```python
from build123d import *

# Parameters (mm, degrees)
F1_DEPTH = 19.05
F2_W     = 152.4
F2_H     = 19.05
F3_DEPTH = 19.051
F4_R     = 12.7
F5_DEPTH = 19.051


with BuildPart() as f1:
    # F0 (on Top) → F1 (new body)
    with BuildSketch(Plane.XY):
        Polygon((341.488764, -53.718452), (318.628764, -53.718452), (318.628764, -2.918452), (341.488764, -2.918452), (341.488764, 30.101548), (-268.111236, 30.101548), (-268.111236, -2.918452), (-245.251236, -2.918452), (-245.251236, -53.718452), (-268.111236, -53.718452), (-268.111236, -86.738452), (-268.111236, -105.788452), (341.488764, -105.788452), (341.488764, -86.738452), align=None)
    extrude(amount=F1_DEPTH)

    # F2 (on face) → F3 (cut, through all)
    with BuildSketch(Plane.XY.offset(19.05)):
        with Locations((-115.711236, -96.263452)):
            Rectangle(F2_W, F2_H)
        with Locations((189.088764, -96.263452)):
            Rectangle(F2_W, F2_H)
    extrude(amount=-F3_DEPTH, mode=Mode.SUBTRACT)

    # F4 (on face) → F5 (cut, through all)
    with BuildSketch(Plane.XY.offset(19.05)):
        with Locations((189.088764, -28.318452)):
            Circle(F4_R)
        with Locations((-115.711236, -28.318452)):
            Circle(F4_R)
    extrude(amount=-F5_DEPTH, mode=Mode.SUBTRACT)


solid = f1.part
```
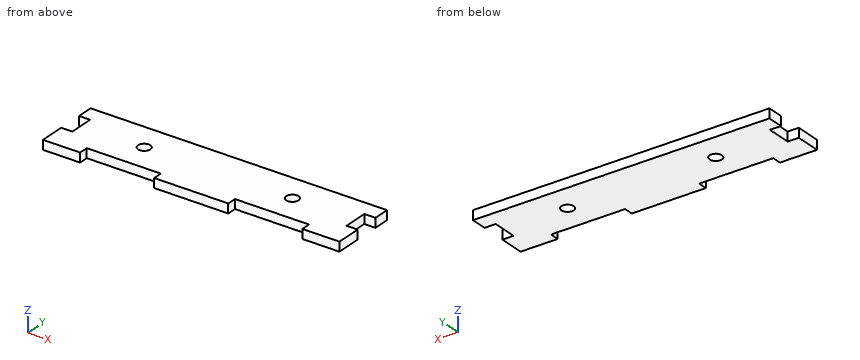
Part model, mm, in its own coordinate system. Coordinates: 2 decimals unless noted, no trailing zeros. Write each loop counter-clockwise with the first axis right and the second up, starting at its lowest first coordinate (ties: lowest second). Pieces come first, ordered by that corner, then holes.
Item 1: Slice it at A-A (x = 190). Write the cut outline in (y, z), and give its area (3 significant figures).
Item 2: Pin check, flat tips, straight feed: pin 1 (5.5 mm diameter, centred on x = -91.5, z = 10.5, fed in from -Y); pin 2 (6 mm diameter, centred on y = -10, z = 16.5, fed in from -X); pin 3 (23 mm diameter, centred on x = -115.71, y = -28.32, fed in from -Z). Stop position of each tip, or through.
Item 3: Probe line 1 (X direction, y = -98, z = 1.5); line 2 (X direction, y = -28, z = 11.75); line 3 (X direction, y = -7.5, z = 13.25). List the from-to ranges inside material, lowest first.
Item 4: Slice it at C-C (y = -10). Write the cut outline in (x, z).
Item 5: Slice it at B-B (z = 5.75). Write the cut outline in (x, y), and give its area (3 significant figures).
Results found:
1. outline: (-86.74, 0) - (-40.99, 0) - (-40.99, 19.05) - (-86.74, 19.05) - close; (-15.65, 0) - (30.1, 0) - (30.1, 19.05) - (-15.65, 19.05) - close
1. area: 1,740 mm2
2. pin 1: stops at y = -86.74
2. pin 2: stops at x = -245.25
2. pin 3: passes through
3. line 1: x = -268.11 to -191.91, -39.51 to 112.89, 265.29 to 341.49
3. line 2: x = -245.25 to -128.41, -103.02 to 176.39, 201.78 to 318.63
3. line 3: x = -245.25 to 318.63
4. outline: (-245.25, 0) - (318.63, 0) - (318.63, 19.05) - (-245.25, 19.05) - close
5. outline: (-268.11, -105.79) - (-191.91, -105.79) - (-191.91, -86.74) - (-39.51, -86.74) - (-39.51, -105.79) - (112.89, -105.79) - (112.89, -86.74) - (265.29, -86.74) - (265.29, -105.79) - (341.49, -105.79) - (341.49, -53.72) - (318.63, -53.72) - (318.63, -2.92) - (341.49, -2.92) - (341.49, 30.1) - (-268.11, 30.1) - (-268.11, -2.92) - (-245.25, -2.92) - (-245.25, -53.72) - (-268.11, -53.72) - close; hole circle Ø25.4 at (-115.71, -28.32); hole circle Ø25.4 at (189.09, -28.32)
5. area: 73,700 mm2
